from build123d import *

# Parameters (mm, degrees)
BOSS_EXTRUDE1_DEPTH     = 10
BOSS_EXTRUDE2_START     = 10
SKETCH1_3_R             = 20
SKETCH1_3_R_2           = 5
BOSS_EXTRUDE2_DEPTH     = 10
SKETCH1_5_R             = 20
BOSS_EXTRUDE3_DEPTH     = 15
CUT_EXTRUDE1_DEPTH      = 215.297519294
CUT_EXTRUDE1_DEPTH_BACK = 215.297519294
SKETCH1_6_R             = 5


with BuildPart() as part:
    # Sketch1 → Boss-Extrude1 (new body)
    with BuildSketch(Plane.XY):
        with BuildLine():
            Line((-32.55466062, 173.476173045), (72.802083582, 173.476173045))
            ThreePointArc((72.802083582, 173.476173045), (79.861224101, 170.559148064), (82.802026774, 163.50988007))
            Line((82.802026774, 163.50988007), (83.39706002, -13.020047424))
            ThreePointArc((83.39706002, -13.020047424), (80.480091848, -20.112894968), (73.397116829, -23.053754449))
            Line((73.397116829, -23.053754449), (-95.173260832, -23.053754449))
            ThreePointArc((-95.173260832, -23.053754449), (-99.882498656, -21.875493456), (-103.481994233, -18.618370272))
            ThreePointArc((-103.481994233, -18.618370272), (-117.625312011, 94.28140669), (-35.49963159, 173.032696784))
            ThreePointArc((-35.49963159, 173.032696784), (-34.043748026, 173.364682472), (-32.55466062, 173.476173045))
        make_face()
    extrude(amount=-BOSS_EXTRUDE1_DEPTH)

    # Sketch1_3 → Boss-Extrude2 (add)
    # profile 1 of 4: a face of its own
    with BuildSketch(Plane.XY.offset(BOSS_EXTRUDE2_START)):
        with BuildLine():
            Line((-32.55466062, 173.476173045), (72.802083582, 173.476173045))
            ThreePointArc((72.802083582, 173.476173045), (79.861224101, 170.559148064), (82.802026774, 163.50988007))
            Line((82.802026774, 163.50988007), (83.39706002, -13.020047424))
            ThreePointArc((83.39706002, -13.020047424), (80.480091848, -20.112894968), (73.397116829, -23.053754449))
            Line((73.397116829, -23.053754449), (-95.173260832, -23.053754449))
            ThreePointArc((-95.173260832, -23.053754449), (-99.882498656, -21.875493456), (-103.481994233, -18.618370272))
            ThreePointArc((-103.481994233, -18.618370272), (-117.625312011, 94.28140669), (-35.49963159, 173.032696784))
            ThreePointArc((-35.49963159, 173.032696784), (-34.043748026, 173.364682472), (-32.55466062, 173.476173045))
        make_face()
        with Locations((50, 1.860098346)):
            Circle(SKETCH1_3_R, mode=Mode.SUBTRACT)
        with Locations((-18.514628019, 72.64435198)):
            Circle(SKETCH1_3_R_2, mode=Mode.SUBTRACT)
        with BuildLine():
            Line((39.999999943, 66.719217535), (39.999999943, 86.719217535))
            ThreePointArc((39.999999943, 86.719217535), (24.076427728, 120.796742868), (-12.279317814, 130.445455266))
            ThreePointArc((-12.279317814, 130.445455266), (-56.931818797, 105.894326865), (-77.620913723, 59.326472063))
            ThreePointArc((-77.620913723, 59.326472063), (-66.565807676, 25.652999614), (-34.394574448, 10.78256354))
            Line((-34.394574448, 10.78256354), (-14.394574448, 10.329008016))
            ThreePointArc((-14.394574448, 10.329008016), (-4.623864336, 0.104858961), (-14.848013391, -9.665851152))
            Line((-14.848013391, -9.665851152), (-34.848013391, -9.212295627))
            ThreePointArc((-34.848013391, -9.212295627), (-81.502346372, 12.352630755), (-97.534327335, 61.185492868))
            ThreePointArc((-97.534327335, 61.185492868), (-71.659502341, 119.425599438), (-15.814833806, 150.130478169))
            ThreePointArc((-15.814833806, 150.130478169), (36.907828278, 136.13803225), (59.999999943, 86.719217535))
            Line((59.999999943, 86.719217535), (59.999999943, 66.719217535))
            ThreePointArc((59.999999943, 66.719217535), (49.999999943, 56.719217535), (39.999999943, 66.719217535))
        make_face(mode=Mode.SUBTRACT)
    # profile 2 of 4: a face of its own
    with BuildSketch(Plane.XY.offset(BOSS_EXTRUDE2_START)):
        with Locations((50, 1.860098346)):
            Circle(SKETCH1_3_R)
        with Locations((50, 1.860098346)):
            Circle(SKETCH1_3_R_2, mode=Mode.SUBTRACT)
    # profile 3 of 4: a face of its own
    with BuildSketch(Plane.XY.offset(BOSS_EXTRUDE2_START)):
        with Locations((50, 1.860098346)):
            Circle(SKETCH1_3_R_2)
    # profile 4 of 4: a face of its own
    with BuildSketch(Plane.XY.offset(BOSS_EXTRUDE2_START)):
        with Locations((-18.514628019, 72.64435198)):
            Circle(SKETCH1_3_R_2)
    extrude(amount=-BOSS_EXTRUDE2_DEPTH)

    # Sketch1_5 → Boss-Extrude3 (add)
    with BuildSketch(Plane.XY):
        with Locations((50, 1.860098346)):
            Circle(SKETCH1_5_R)
    extrude(amount=BOSS_EXTRUDE3_DEPTH)

    # Sketch1_6 → Cut-Extrude1 (cut, two sides: drawn at the far end of the back side and taken through both)
    with BuildSketch(Plane.XY.offset(-CUT_EXTRUDE1_DEPTH_BACK)):
        with Locations((-18.514628019, 72.64435198)):
            Circle(SKETCH1_6_R)
        with Locations((50, 1.860098346)):
            Circle(SKETCH1_6_R)
    extrude(amount=CUT_EXTRUDE1_DEPTH + CUT_EXTRUDE1_DEPTH_BACK, mode=Mode.SUBTRACT)


solid = part.part
Source: CAD feature listing. Evaluate the final solid. Frame: model axes, mm. A direction names the side the tool comes from. Round coordinates to 2 decimals unless told otherwise and drop trailing zeros. Write each loop counter-clockwise with the first axis right and the second up, starting at its lowest first coordinate (ties: lowest second). Pieces come first, ordered by that corner, then holes. Notation, with made-up numbers: M -36.75,-13 L 6.25,-13 A20 cw 6.25,11 Z; hole C 60.25,28 d3. An arc over 180 degrees is marked long. One line per item, written item: value. Start each with the question number.
Item 1: Section query A-A (x = 50). Return the cut outline in (y, z).
Item 2: Pin query (flat end, axial travel): pin 1 (6 mm diameter, centred on x = -59, y = 126, fed in from +Z); pin 2 (2 mm diameter, centred on y = 83.5, z = -2, fed in from -X); pin 3 (6 mm diameter, centred on x = 26.5, y = 0, fed in from +Z). Return the tip coordinate at first contact, or that it passes through.
Item 3: Ray query, L1, parallel to Y at x = 50, z = 1.25; L2, parallel to Z at x = 13, y = 89; L3, parallel to Y at x = 31.5, z = 9. Return the intervals inside material, ascending. Write a range as from..to.
Item 4: Section query D-D (x = 18.5). Return the cut outline in (y, z).
Item 5: Section query B-B (y = 125). Return the cut outline in (x, z), plus the area to 3 significant figures.
Item 6: Set-up query: faces 1 (the cylindrical face through (-66.903, 26.036, 5.07)), 2 (the flat face through (54, -2, 15)). Return all of +Z, -Z, +X, -X, +Y, -Y with unobstructed straight access to the full face (end or side cutting, diameter ignored); none if empty.
Item 7: Section query C-C (z = 7). Return the cut outline in (x, y), plus the area to 3 significant figures.
Item 8: Mould query, pull axis Y, two halves, no side actions, for faces 3 (the flat face through (40, 77, 5)), 4 (the flat face through (19, 173.476, 0)), 5 (the flat face through (-10, -23.054, 0)). Classes: pulls with the +Y half, pulls with the -Y half, needs draft (parallel to the pull), parting line crosses it, or undercut.
Result set:
1. outline: M -23.05,-10 L -3.14,-10 L -3.14,15 L -18.14,15 L -18.14,10 L -23.05,10 Z; M 6.86,-10 L 173.48,-10 L 173.48,10 L 121.19,10 L 121.19,0 L 56.72,0 L 56.72,10 L 21.86,10 L 21.86,15 L 6.86,15 Z
2. pin 1: stops at z = 0
2. pin 2: stops at x = -121.17
2. pin 3: stops at z = 10
3. L1: y = -23.05..-3.14, 6.86..56.72, 121.19..173.48
3. L2: z = -10..10
3. L3: y = -23.05..112.85, 140.2..173.48
4. outline: M -23.05,-10 L 173.48,-10 L 173.48,10 L 146.93,10 L 146.93,0 L 124.77,0 L 124.77,10 L -23.05,10 Z
5. outline: M -101.72,-10 L 82.93,-10 L 82.93,10 L 47.39,10 L 47.39,0 L 18.12,0 L 18.12,10 L -30.18,10 L -30.18,0 L -66.12,0 L -66.12,10 L -101.72,10 Z
5. area: 3,040 mm²
6. face 1: +Z
6. face 2: +Z, +X, -X, +Y, -Y
7. outline: M -103.48,-18.62 A10 ccw -95.17,-23.05 L 73.4,-23.05 A10 ccw 83.4,-13.02 L 82.8,163.51 A10 ccw 72.8,173.48 L -32.55,173.48 A10 ccw -35.5,173.03 A126.74 ccw Z; hole M -97.53,61.19 A64.43 ccw -34.85,-9.21 L -14.85,-9.67 A10 ccw -14.39,10.33 L -34.39,10.78 A44.43 cw -77.62,59.33 A79.79 cw -12.28,130.45 A44.43 cw 40,86.72 L 40,66.72 A10 ccw 60,66.72 L 60,86.72 A64.43 ccw -15.81,150.13 A99.79 ccw Z; hole C -18.51,72.64 d10; hole C 50,1.86 d10
7. area: 30,000 mm²
8. face 3: undercut
8. face 4: pulls with the +Y half
8. face 5: pulls with the -Y half
